Read the model definition and answer for the solid it produces. Units are mm, in the model's axes. Give positions to 0.01 mm unless a question says otherwise; leave off trailing zeros. Write each loop counter-clockwise with the first axis right and the second up, starting at its lowest first coordinate (ties: lowest second). Pieces come first, ordered by that corner, then holes. Notation, with made-up numbers: (43.25, -35.5) -> (86.25, -35.5) arc R12 ccw to (86.25, -29.5) -> close; hole circle Ø7 at (76, 83). An arc over 180 degrees is marked (long way). Answer as CSV lines item,"result". Start each with the question number.
1. The part is cut by section C-C, the plane x = -17.5. Determine the outline of the cut face in (y, z) (3 decimals), and give its area (3 significant figures).
2. Given pin 1 (7.5 mm diameter, centred on x = -17.46, y = -12.7, fed in from -Z); pin 2 (1 mm diameter, centred on x = -2.5, z = 2, fed in from -Y); pin 3 (4 mm diameter, centred on x = -17.46, y = -47.62, fed in from +Z); pin 4 (1 mm diameter, centred on x = 37, y = -13, fed in from +Z), each flat-ended and moving along its own axis, determine where each tip first touches the part or whether it passes through.
3. For a pull along X with two mould halves and no side action, classify faces 1 (the cylindrical face through (-3.21, -1.587, 1.609)), 2 (the flat face through (-38, -60.325, 2)), 3 (the flat face through (114.3, -30, 2)), 4 (the flat face through (-69.85, -30, 2)) as pulls with the +X half, pulls with the -X half, needs draft (parallel to the pull), parting line crosses it, or undercut.
4. The part is cut by section A-A, the plane x = 102.87. Determine the outline of the cut face in (y, z) (3 decimals).
5. The part is cut by section B-B, the plane y = -12.7. Give the number of separate pieces and of enclosed holes in the cut face, and give its area (3 significant figures).
6. Find the intervals of material crossed by line 1 (Y direction, x = 102.87, z = 1.6) (3 decimals); line 2 (Y direction, x = -57.15, z = 1.1) (3 decimals); line 3 (X direction, y = -13, z = 0.4), in increasing order.
from build123d import *

# Parameters (mm, degrees)
F1_DEPTH = 60.325
F2_R     = 8.001
F3_DEPTH = 25.4
F4_R     = 3.175
F5_DEPTH = 25.4
F6_R     = 3.175
F7_DEPTH = 25.4
F9_DEPTH = 25.4


with BuildPart() as f1:
    # F0 (on Front) → F1 (new body)
    with BuildSketch(Plane.XZ):
        Polygon((-4.7625, 3.175), (-69.85, 3.175), (-69.85, 0), (-4.7625, 0), (70.1675, -0.0282659046), (114.3, -0.0282659046), (114.3, 3.1467340954), (70.1675, 3.1467340954), align=None)
    extrude(amount=F1_DEPTH)

    # F2 (on face) → F3 (cut)
    with BuildSketch(Plane.XY.offset(3.1467340954)):
        with Locations((102.87, -12.7)):
            Circle(F2_R)
        with Locations((102.87, -47.625)):
            Circle(F2_R)
    extrude(amount=-F3_DEPTH, mode=Mode.SUBTRACT)

    # F4 (on face) → F5 (cut)
    with BuildSketch(Plane.XY.offset(3.175)):
        with Locations((-57.15, -12.7)):
            Circle(F4_R)
        with Locations((-57.15, -47.625)):
            Circle(F4_R)
    extrude(amount=-F5_DEPTH, mode=Mode.SUBTRACT)

    # F6 (on face) → F7 (cut)
    with BuildSketch(Plane.XY.offset(3.175)):
        with Locations((-17.4625, -12.7)):
            Circle(F6_R)
        with Locations((-17.4625, -47.625)):
            Circle(F6_R)
    extrude(amount=-F7_DEPTH, mode=Mode.SUBTRACT)

    # F8 (on face) → F9 (cut)
    with BuildSketch(Plane(origin=(0.0011970299, 0, 3.1732029867), x_dir=(0.9999999288, 0, -0.0003772308), z_dir=(0.0003772308, 0, 0.9999999288))):
        with BuildLine():
            ThreePointArc((-1.5886973689, -60.325), (-3.1761973689, -58.7375), (-4.7636973689, -60.325))
            Line((-4.7636973689, -60.325), (-1.5886973689, -60.325))
        make_face()
        with BuildLine():
            ThreePointArc((70.1663079625, -60.325), (68.5788079625, -58.7375), (66.9913079625, -60.325))
            Line((66.9913079625, -60.325), (70.1663079625, -60.325))
        make_face()
        with BuildLine():
            Line((70.1663079625, 0), (66.9913079625, 0))
            ThreePointArc((66.9913079625, 0), (68.5788079625, -1.5875), (70.1663079625, 0))
        make_face()
        with BuildLine():
            Line((-1.5886973689, 0), (-4.7636973689, 0))
            ThreePointArc((-4.7636973689, 0), (-3.1761973689, -1.5875), (-1.5886973689, 0))
        make_face()
    extrude(amount=-F9_DEPTH, mode=Mode.SUBTRACT)


solid = f1.part
Results found:
1,outline,"(-60.325, 0) -> (-50.8, 0) -> (-50.8, 3.175) -> (-60.325, 3.175) -> close; (-44.45, 0) -> (-15.875, 0) -> (-15.875, 3.175) -> (-44.45, 3.175) -> close; (-9.525, 0) -> (0, 0) -> (0, 3.175) -> (-9.525, 3.175) -> close"
1,area,"151 mm²"
2,pin 1,"stops at z = 0"
2,pin 2,"stops at y = -59.26"
2,pin 3,"passes through"
2,pin 4,"stops at z = 3.16"
3,face 1,"undercut"
3,face 2,"needs draft"
3,face 3,"pulls with the +X half"
3,face 4,"pulls with the -X half"
4,outline,"(-60.325, -0.028) -> (-55.626, -0.028) -> (-55.626, 3.147) -> (-60.325, 3.147) -> close; (-39.624, -0.028) -> (-20.701, -0.028) -> (-20.701, 3.147) -> (-39.624, 3.147) -> close; (-4.699, -0.028) -> (0, -0.028) -> (0, 3.147) -> (-4.699, 3.147) -> close"
5,separate pieces,"4"
5,enclosed holes,"0"
5,area,"494 mm²"
6,line 1,"y = -60.325 to -55.626, -39.624 to -20.701, -4.699 to 0"
6,line 2,"y = -60.325 to -50.8, -44.45 to -15.875, -9.525 to 0"
6,line 3,"x = -69.85 to -60.31, -53.99 to -20.62, -14.3 to 94.87, 110.87 to 114.3"
